from build123d import *

# Parameters (mm, degrees)
BOSS_EXTRUDE2_DEPTH = 6.35
CIRPATTERN8_COUNT   = 2
SKETCH17_R          = 5.08
BOSS_EXTRUDE3_DEPTH = 6.35
SKETCH18_R          = 2.54
BOSS_EXTRUDE4_DEPTH = 6.35


with BuildPart() as part:
    # Sketch16 → Boss-Extrude2 (new body)
    with BuildSketch(Plane(origin=(0, 0, 0), x_dir=(1, 0, 0), z_dir=(0, 1, 0))):
        Polygon((34.18332, 3.175), (0, 3.175), (0, 0), (0, -3.175), (34.18332, -3.175), align=None)
        Polygon((46.453207734, -3.175), (34.18332, -3.175), (34.18332, 3.175), (40.53332, 4.351902935), (39.226311646, 11.403888956), (45.06457303, 12.485946745), (46.453207734, 4.99354435), align=None)
    boss_extrude2 = extrude(amount=BOSS_EXTRUDE2_DEPTH)

    # CirPattern8: Boss-Extrude2 ×2 about axis
    cirpattern8_axis = Axis((0, 0, 0), (0, 1, 0))
    for i in range(1, CIRPATTERN8_COUNT):
        add(boss_extrude2.rotate(cirpattern8_axis, i * 360 / CIRPATTERN8_COUNT))

    # Sketch17 → Boss-Extrude3 (add)
    with BuildSketch(Plane(origin=(0, 0, 0), x_dir=(1, 0, 0), z_dir=(0, 1, 0))):
        with Locations(Location((0, 0, 0), (0, 0, 270))):
            Circle(SKETCH17_R)
    extrude(amount=-BOSS_EXTRUDE3_DEPTH)

    # Sketch18 → Boss-Extrude4 (add)
    with BuildSketch(Plane.XZ.offset(6.35)):
        with Locations(Location((0, 0, 0), (0, 0, 270))):
            Circle(SKETCH18_R)
    extrude(amount=BOSS_EXTRUDE4_DEPTH)


solid = part.part
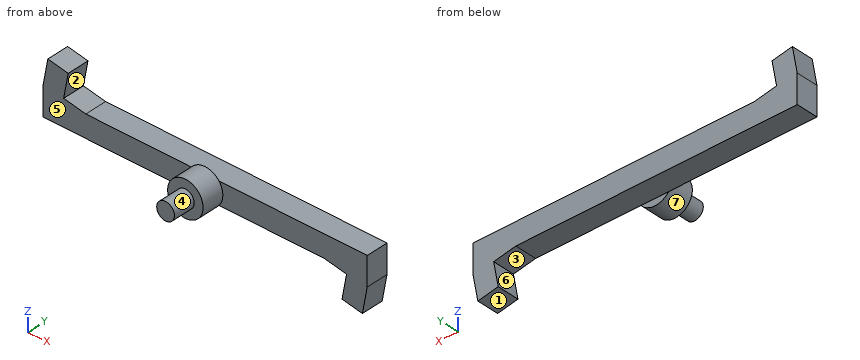
The listing builds one solid part. Answer for the finished solid, in the listing's coordinates (mm). Face numbers are marked on the shaded views. A direction names the side the tool comes from. Coordinates: 2 decimals unless noted, no trailing zeros. Write each loop counter-clockwise with the first axis right and the second up, starting at its lowest first coordinate (ties: lowest second). Pieces come first, ordered by that corner, then holes. Notation, with made-up numbers: M 63,-24.75 L 110,-24.75 A16 cw 110,-7.75 Z; hole C -20.5,-26 d10. An arc over 180 degrees is marked long. Use one line per item in the form item = value.
Item 1: Find section A-A, the plane x = 0. Give the vertices of the cut face in (y, z) (3 decimals), plus the area to 3 significant figures.
Model answer:
outline = M -12.7,-2.54 L -6.35,-2.54 L -6.35,-5.08 L 0,-5.08 L 0,-3.175 L 6.35,-3.175 L 6.35,3.175 L 0,3.175 L 0,5.08 L -6.35,5.08 L -6.35,2.54 L -12.7,2.54 Z
area = 137 mm2
Item 2: Find section C-C, the plane y = -10.25. Give the vertices of the cut face in (x, z).
Model answer:
outline = C 0,0 d5.08
Item 3: The mould has two halves that part along Z. Classify the marked faces 5, 6 and 7: released by +Z, released by -Z, zero draft, split by the parting line, or undercut.
Model answer:
face_5 = zero draft
face_6 = undercut
face_7 = split by the parting line
Item 4: Find section D-D, the plane y = -3.5. Give the vertices of the cut face in (x, z).
Model answer:
outline = C 0,0 d10.16
Item 5: Find section B-B, the plane z = 0. Give the vertices of the cut face in (x, y), plus the area to 3 significant figures.
Model answer:
outline = M -46.45,0 L -5.08,0 L -5.08,-6.35 L -2.54,-6.35 L -2.54,-12.7 L 2.54,-12.7 L 2.54,-6.35 L 5.08,-6.35 L 5.08,0 L 46.45,0 L 46.45,6.35 L -46.45,6.35 Z
area = 687 mm2
Item 6: Given P1, Ø12.5, axis at x = 35.5, z = -3, coming from the -Y side; P2, Ø1.5, axis at x = 1.5, z = -4, coming from the +Y side; P3, Ø5, axis at x = -6.5, y = 3, coming from the +Z side (3 decimals), each flat-ended and moving along its own axis, determine where each tip first touches the part or whether it passes through.
Model answer:
P1 = 0
P2 = 0
P3 = 3.175
Item 7: Find the intervals of material crossed by probe 1 along X at (y, z) = (-2, 0); probe 2 along Z at (x, y) = (25, 2.75) (3 decimals); probe 3 along Y at (x, z) = (-31.5, -2.5), in increasing order.
Model answer:
probe_1 = -5.08 to 5.08
probe_2 = -3.175 to 3.175
probe_3 = 0 to 6.35
Item 8: For the marked faces 1, 2, 3 and 4, determine the directions among +Z, -Z, +X, -X, +Y, -Y from which every point of the face is accessible in a straight line to the end or side of a thin tool.
Model answer:
face_1 = -Z, -X, +Y, -Y
face_2 = +X, +Y, -Y
face_3 = -X, +Y, -Y
face_4 = -Y
